from build123d import *

# Parameters (mm, degrees)
SKETCH_1_W          = 40
SKETCH_1_H          = 40
SKETCH_1_W_2        = 38
SKETCH_1_H_2        = 38
EXTRUDE_1_DEPTH     = 295
SKETCH_2_R          = 1.6
CUT_EXTRUDE_1_DEPTH = 299.370574957


with BuildPart() as part:
    # 草图1 → 凸台-拉伸1 (new, symmetric)
    with BuildSketch(Plane.XY):
        Rectangle(SKETCH_1_W, SKETCH_1_H)
        Rectangle(SKETCH_1_W_2, SKETCH_1_H_2, mode=Mode.SUBTRACT)
    extrude(amount=EXTRUDE_1_DEPTH, both=True)

    # 草图2 → 切除-拉伸1 (cut, through all)
    with BuildSketch(Plane(origin=(0, 20, 0), x_dir=(1, 0, 0), z_dir=(0, 1, 0))):
        with Locations(Location((-10, -285, 0), (0, 0, 270))):
            Circle(SKETCH_2_R)
        with Locations(Location((10, -285, 0), (0, 0, 270))):
            Circle(SKETCH_2_R)
        with Locations(Location((-10, -265, 0), (0, 0, 270))):
            Circle(SKETCH_2_R)
        with Locations(Location((10, -265, 0), (0, 0, 270))):
            Circle(SKETCH_2_R)
        with Locations(Location((-10, -245, 0), (0, 0, 270))):
            Circle(SKETCH_2_R)
        with Locations(Location((10, -245, 0), (0, 0, 270))):
            Circle(SKETCH_2_R)
        with Locations(Location((-10, -225, 0), (0, 0, 270))):
            Circle(SKETCH_2_R)
        with Locations(Location((10, -225, 0), (0, 0, 270))):
            Circle(SKETCH_2_R)
        with Locations(Location((10, 225, 0), (0, 0, 270))):
            Circle(SKETCH_2_R)
        with Locations(Location((-10, 225, 0), (0, 0, 270))):
            Circle(SKETCH_2_R)
        with Locations(Location((10, 245, 0), (0, 0, 270))):
            Circle(SKETCH_2_R)
        with Locations(Location((-10, 245, 0), (0, 0, 270))):
            Circle(SKETCH_2_R)
        with Locations(Location((10, 265, 0), (0, 0, 270))):
            Circle(SKETCH_2_R)
        with Locations(Location((-10, 265, 0), (0, 0, 270))):
            Circle(SKETCH_2_R)
        with Locations(Location((10, 285, 0), (0, 0, 270))):
            Circle(SKETCH_2_R)
        with Locations(Location((-10, 285, 0), (0, 0, 270))):
            Circle(SKETCH_2_R)
    extrude(amount=-CUT_EXTRUDE_1_DEPTH, mode=Mode.SUBTRACT)


solid = part.part
Model file for the job. Use its own axes, mm. A direction names the side the tool comes from. Give positions to 0.01 mm unless a question says otherwise; leave off trailing zeros. Order: outer loops, then holes, each group sorted by start corner. A loop starts at its lowest first (then second) coordinate and runs counter-clockwise, first axis right, second up. Notation, with made-up numbers: (75, 30) - (116, 30) arc R21 cw to (116, 35) - close; hole circle Ø7 at (39.25, 85.25). An arc over 180 degrees is marked (long way). Return JSON: item names as keys, results as strings.
1) 3-axis set-ups, long thin cutter, end or side, ignore diameter. For faces 5 (the flat face through (-19, 0, 4)), 6 (the flat face through (-1.6, -19.2, 295)): which of +Z, -Z, +X, -X, +Y, -Y reach the whole face in a straight line?
Geometry says:
{"face 5": "+Z, -Z", "face 6": "+Z, +X, -X, +Y, -Y"}
2) Pull direction Y, two halves, no side cores. Call faces 1 (the flat face through (0, -19, 4)), 2 (the flat face through (-1.6, -19.2, -295)), 3 (the flat face through (0, 19, 4)), 4 (the flat face through (0, 20, 4)): pulls with the +Y half, pulls with the -Y half, needs draft (parallel to the pull), parting line crosses it, or undercut.
Geometry says:
{"face 1": "undercut", "face 2": "needs draft", "face 3": "undercut", "face 4": "pulls with the +Y half"}
3) Cut at C-C, the plane z = -154.5. Give the cut face in (x, y), plus the area to 3 significant figures.
Geometry says:
{"outline": "(-20, -20) - (20, -20) - (20, 20) - (-20, 20) - close; hole (-19, -19) - (19, -19) - (19, 19) - (-19, 19) - close", "area": "156 mm²"}
4) Cut at A-A, the plane x = 3. Give the cut face in (y, z).
Geometry says:
{"outline": "(-20, -295) - (-19, -295) - (-19, 295) - (-20, 295) - close; (19, -295) - (20, -295) - (20, 295) - (19, 295) - close"}
5) Probe line 1 (X direction, y = 19.8, z = 225); line 2 (Y direction, x = -15, z = -99.5). List the from-to ranges inside material, lowest first. Write a range as from..to.
Geometry says:
{"line 1": "-20..-11.6, -8.4..8.4, 11.6..20", "line 2": "-20..-19, 19..20"}
